Design review of the part built by this model. Coordinates are the model's own, in mm. A direction names the side the tool comes from. Coordinates: 2 decimals unless noted, no trailing zeros. Order: outer loops, then holes, each group sorted by start corner. A loop starts at its lowest first (then second) coordinate and runs counter-clockwise, first axis right, second up.
from build123d import *

# Parameters (mm, degrees)
F1_DEPTH = 25


with BuildPart() as f1:
    # F0 (on Front) → F1 (new body)
    with BuildSketch(Plane.XZ):
        with BuildLine():
            Line((-1.422933, 10.220143), (1.327067, 10.220143))
            Line((1.327067, 10.220143), (6.327067, 10.220143))
            Line((6.327067, 10.220143), (6.327067, 10.027808))
            ThreePointArc((6.327067, 10.027808), (9.535739, 14.190085), (10.677067, 19.320143))
            ThreePointArc((10.677067, 19.320143), (10.621655, 20.476818), (10.455927, 21.622899))
            Line((10.455927, 21.622899), (7.380891, 21.622899))
            ThreePointArc((7.380891, 21.622899), (7.602719, 20.481005), (7.677067, 19.320143))
            ThreePointArc((7.677067, 19.320143), (5.011739, 12.885472), (-1.422933, 10.220143))
        make_face()
        with BuildLine():
            ThreePointArc((-9.172933, 10.027808), (-6.818653, 8.489806), (-4.172933, 7.536787))
            Line((-4.172933, 7.536787), (-4.172933, 10.220143))
            Line((-4.172933, 10.220143), (-9.172933, 10.220143))
            Line((-9.172933, 10.220143), (-9.172933, 10.027808))
        make_face()
        with BuildLine():
            ThreePointArc((-4.172933, 7.536787), (-2.807018, 7.299565), (-1.422933, 7.220143))
            ThreePointArc((-1.422933, 7.220143), (-0.038848, 7.299565), (1.327067, 7.536787))
            Line((1.327067, 7.536787), (1.327067, 10.220143))
            Line((1.327067, 10.220143), (-1.422933, 10.220143))
            Line((-1.422933, 10.220143), (-4.172933, 10.220143))
            Line((-4.172933, 10.220143), (-4.172933, 7.536787))
        make_face()
        with BuildLine():
            Line((1.327067, 10.220143), (1.327067, 7.536787))
            ThreePointArc((1.327067, 7.536787), (3.972787, 8.489806), (6.327067, 10.027808))
            Line((6.327067, 10.027808), (6.327067, 10.220143))
            Line((6.327067, 10.220143), (1.327067, 10.220143))
        make_face()
        with BuildLine():
            Line((1.327067, 7.536787), (1.327067, 7.220143))
            Line((1.327067, 7.220143), (1.327067, -9.779857))
            Line((1.327067, -9.779857), (6.327067, -9.779857))
            Line((6.327067, -9.779857), (6.327067, 10.027808))
            ThreePointArc((6.327067, 10.027808), (3.972787, 8.489806), (1.327067, 7.536787))
        make_face()
        with BuildLine():
            ThreePointArc((1.327067, 7.536787), (-0.038848, 7.299565), (-1.422933, 7.220143))
            Line((-1.422933, 7.220143), (1.327067, 7.220143))
            Line((1.327067, 7.220143), (1.327067, 7.536787))
        make_face()
        with BuildLine():
            Line((-4.172933, 7.536787), (-4.172933, 7.220143))
            Line((-4.172933, 7.220143), (-1.422933, 7.220143))
            ThreePointArc((-1.422933, 7.220143), (-2.807018, 7.299565), (-4.172933, 7.536787))
        make_face()
        with BuildLine():
            Line((-4.172933, -9.779857), (-4.172933, 7.220143))
            Line((-4.172933, 7.220143), (-4.172933, 7.536787))
            ThreePointArc((-4.172933, 7.536787), (-6.818653, 8.489806), (-9.172933, 10.027808))
            Line((-9.172933, 10.027808), (-9.172933, -9.779857))
            Line((-9.172933, -9.779857), (-4.172933, -9.779857))
        make_face()
        with BuildLine():
            Line((-9.172933, 10.220143), (-4.172933, 10.220143))
            Line((-4.172933, 10.220143), (-1.422933, 10.220143))
            ThreePointArc((-1.422933, 10.220143), (-8.625886, 13.758897), (-10.226757, 21.622899))
            Line((-10.226757, 21.622899), (-13.301793, 21.622899))
            ThreePointArc((-13.301793, 21.622899), (-12.821818, 15.26115), (-9.172933, 10.027808))
            Line((-9.172933, 10.027808), (-9.172933, 10.220143))
        make_face()
    extrude(amount=F1_DEPTH)


solid = f1.part
1. To check wall thickness, follow line 1 (X direction, y = -0.75, z = -8); line 2 (X direction, y = -13, z = 19.5); line 3 (Z direction, x = -4.25, y = -10). State the ranges of each line that lie inside material, in increasing order.
2. Insertion check: pin 1 (12 mm diameter, centred on y = -20, z = 2.5, fed in from -X); pin 2 (6 mm diameter, centred on y = -9.5, z = 0, fed in from +X); pin 3 (1 mm diameter, centred on x = -2, y = -22.5, fed in from +Z). Each pin has a flat end and moves straight along its axis. Give the tip position at first contact, or say it passes through.
3. For faces 1 (the flat face through (6.327, -12, 0)), 2 (the flat face through (-9.173, -12, 0)), 3 (the flat face through (-1, -12, 7.22)), list the 3-axis set-ups (+Z, -Z, +X, -X, +Y, -Y) from which the entire face can be reached by the end or side of a thin tool; tool diameter is ignored.
4. Add section A-A (z = -0.5). Give the boundary of the cut face in (x, y), and give its area (3 significant figures).
5. Add section D-D (x = -12). Give the boundary of the cut face in (y, z).
6. Add section C-C (z = 17). Give the boundary of the cut face in (x, y), and give its area (3 significant figures).
7. Add section B-B (y = -19.25). Give the boundary of the cut face in (x, z).
8. Mouldability with a two-part tool opening along X and no side actions: class faces 4 (the flat face through (-4.173, -12, -1)), 5 (the flat face through (1.327, -12, -1)), 6 (the cylindrical face through (9.504, -12.325, 14.123)), 7 (the flat face through (-1, 0, 8)) as pulls with the +X half, pulls with the -X half, needs draft (parallel to the pull), parting line crosses it, or undercut.
Solution:
1. line 1: x = -9.17 to -4.17, 1.33 to 6.33
1. line 2: x = -13.52 to -10.52, 7.68 to 10.68
1. line 3: z = -9.78 to 10.67
2. pin 1: stops at x = -9.17
2. pin 2: stops at x = 6.33
2. pin 3: stops at z = 10.28
3. face 1: -Z, +X, +Y, -Y
3. face 2: -Z, -X, +Y, -Y
3. face 3: -Z, +Y, -Y
4. outline: (-9.17, -25) - (-4.17, -25) - (-4.17, 0) - (-9.17, 0) - close; (1.33, -25) - (6.33, -25) - (6.33, 0) - (1.33, 0) - close
4. area: 250 mm2
5. outline: (-25, 13.44) - (0, 13.44) - (0, 21.62) - (-25, 21.62) - close
6. outline: (-13.3, -25) - (-10.22, -25) - (-10.22, 0) - (-13.3, 0) - close; (7.38, -25) - (10.45, -25) - (10.45, 0) - (7.38, 0) - close
6. area: 154 mm2
7. outline: (-13.3, 21.62) arc R12.1 ccw to (-9.17, 10.03) - (-9.17, -9.78) - (-4.17, -9.78) - (-4.17, 7.22) - (1.33, 7.22) - (1.33, -9.78) - (6.33, -9.78) - (6.33, 10.03) arc R12.1 ccw to (10.68, 19.32) arc R12.1 ccw to (10.46, 21.62) - (7.38, 21.62) arc R9.1 cw to (7.68, 19.32) arc R9.1 cw to (-1.42, 10.22) arc R9.1 cw to (-10.23, 21.62) - close
8. face 4: undercut
8. face 5: undercut
8. face 6: pulls with the +X half
8. face 7: needs draft
